Autodesk Inventor part; units mm, degrees
ref_plane "YZ Plane" through (0, 0, 0) normal (1, 0, 0) x (0, 1, 0)
ref_plane "XZ Plane" through (0, 0, 0) normal (0, 1, 0) x (-1, 0, 0)
ref_plane "XY Plane" through (0, 0, 0) normal (0, 0, 1) x (1, 0, 0)
sketch "Sketch2" plane through (0, 0, 0) normal (0, 1, 0) x (-1, 0, 0)
  line L0 (0, 0) -> (0, -7.9375)
  line L1 (0, -7.9375) -> (9.525, -7.9375)
  line L2 (9.525, -7.9375) -> (9.525, -1.5875)
  line L3 (9.525, -1.5875) -> (3.175, -4.7625)
  line L4 (3.175, -4.7625) -> (3.175, 0)
  line L5 (3.175, 0) -> (0, 0)
  line L6 (0, 0) -> (0, 7.9375)
  line L7 (0, 7.9375) -> (9.525, 7.9375)
  line L8 (9.525, 7.9375) -> (9.525, 1.5875)
  line L9 (9.525, 1.5875) -> (3.175, 4.7625)
  line L10 (3.175, 4.7625) -> (3.175, 0)
  dimension "d1" = 7.9375
  dimension "d2" = 9.525
  dimension "d3" = 6.35
  dimension "d4" = 4.7625
  dimension "d5" = 3.175
extrude "Extrusion1" add sketch "Sketch2" along normal mid plane 50.8
properties part number "testcombine"
Could you check a few things on this model? Use its own coordinates, in mm. A direction names the side the tool comes from. Coordinates: 2 decimals unless noted, no trailing zeros. Loops run counter-clockwise (first coordinate to the right, second up) from the corner with the lowest first, then second, coordinate; pieces in that order, holes last.
1. Imagine slicing it at D-D (z = -0.75). Please give me the cut outline in (x, y) (3 decimals), and give its area (3 significant figures).
2. Imagine slicing it at A-A (x = -7). Please give me the cut outline in (y, z), and give its area (3 significant figures).
3. I need wall thicknesses on L1, parallel to X at y = 14, z = 1 (3 decimals); L2, parallel to X at y = 13.5, z = -2.75 (3 decimals); L3, parallel to X at y = 17.5, z = 3 (3 decimals). Which ranges of each line are inside material? Lowest first, please.
4. We'd pull the mould along Z, two halves only. Please class faces 3 (the face through (-5, 0, -7.938)), 4 (the face through (-6.394, -0.356, -3.153)), 5 (the face through (-3, 25.4, 0)), 6 (the face through (-6.394, -0.356, 3.153)): released by +Z, released by -Z, zero draft, split by the parting line, or undercut.
5. For faces 1 (the face through (-9.525, 0, 5)), 2 (the face through (-3.175, 0, 0)), which set-ups out of +Z, -Z, +X, -X, +Y, -Y let a thin tool reach every point of the face, with its end or its side?
6. Imagine slicing it at C-C (y = -18). Please give me the cut outline in (x, z) (1 decimal).
7. Imagine slicing it at B-B (z = 4.25). Please give me the cut outline in (x, y) (3 decimals).
Computed values:
1. outline: (-3.175, -25.4) - (0, -25.4) - (0, 25.4) - (-3.175, 25.4) - close
1. area: 161 mm2
2. outline: (-25.4, -7.94) - (25.4, -7.94) - (25.4, -2.85) - (-25.4, -2.85) - close; (-25.4, 2.85) - (25.4, 2.85) - (25.4, 7.94) - (-25.4, 7.94) - close
2. area: 517 mm2
3. L1: x = -3.175 to 0
3. L2: x = -9.525 to -7.2, -3.175 to 0
3. L3: x = -9.525 to -6.7, -3.175 to 0
4. face 3: released by -Z
4. face 4: undercut
4. face 5: zero draft
4. face 6: undercut
5. face 1: +Z, -Z, -X, +Y, -Y
5. face 2: +Y, -Y
6. outline: (-9.5, -7.9) - (0, -7.9) - (0, 7.9) - (-9.5, 7.9) - (-9.5, 1.6) - (-3.2, 4.8) - (-3.2, -4.8) - (-9.5, -1.6) - close
7. outline: (-9.525, -25.4) - (-4.2, -25.4) - (-4.2, 25.4) - (-9.525, 25.4) - close; (-3.175, -25.4) - (0, -25.4) - (0, 25.4) - (-3.175, 25.4) - close
